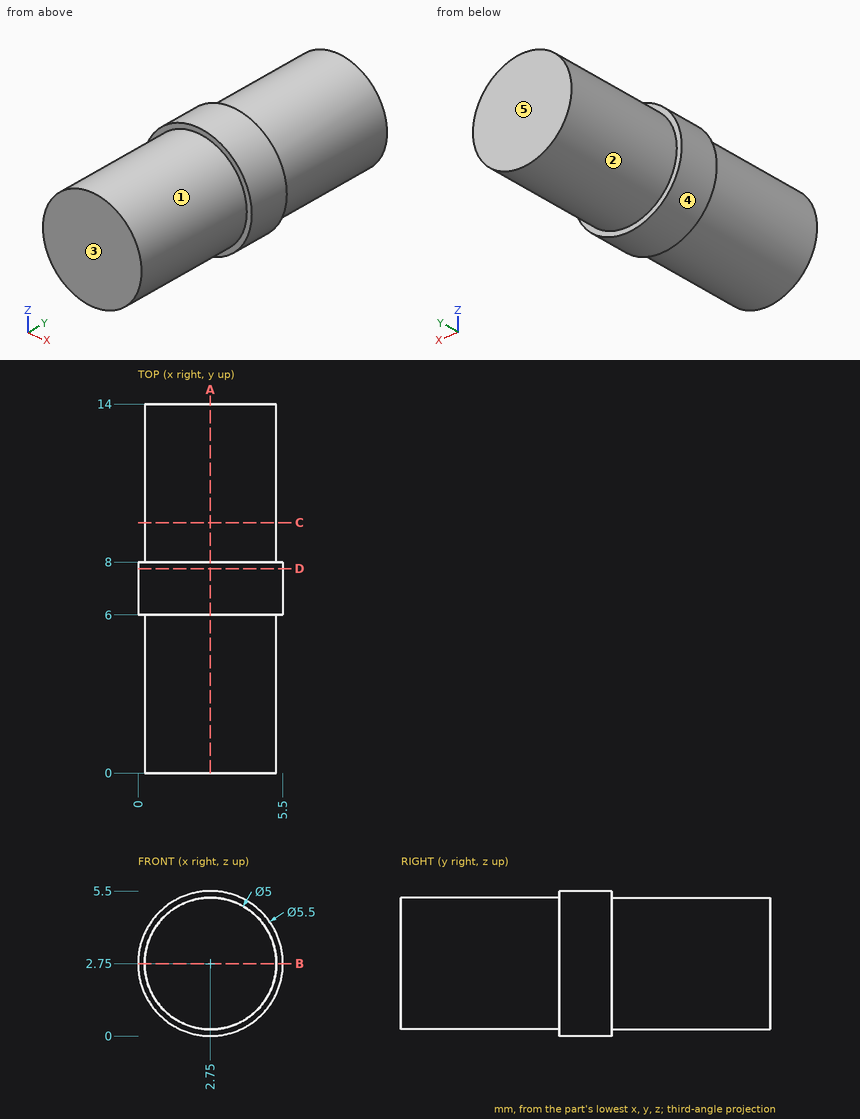
Verification items for this drawing (mm, ordinates from the low corner). A direction names the side the tool comes from. Give positions to 0.01 mm unless a question says otherwise; leave off trailing zeros. Loops run counter-clockwise (first coordinate to the right, second up) from the corner with the lowest first, then second, coordinate; pieces in that order, holes last. Notation, with made-up numbers: M 50.5,-18 L 65.5,-18 A18 ccw 65.5,-4 Z; hole C -19,49 d7. An arc over 180 degrees is marked long. Answer in a Markdown table with one row per item.
1) Tool access check on the marked faces 1, 2 and 3. Record the directions out of +Z, -Z, +X, -X, +Y, -Y that give a thin tool (end or side, any length) a straight path to the whole face; none if there is none.
Solutions:
| item | result |
|---|---|
| face 1 | -Y |
| face 2 | +Y |
| face 3 | +Z, -Z, +X, -X, -Y |
2) Mould release check, pull along Z, two halves, no side actions. Record for the marked faces 4 and 5: released by +Z, released by -Z, zero draft, split by the parting line, or undercut.
Solutions:
| item | result |
|---|---|
| face 4 | split by the parting line |
| face 5 | zero draft |
3) Cross-section at A-A (x = 2.75). Enter the section's corners in (y, z), plus the area to 3 significant figures.
Solutions:
| item | result |
|---|---|
| outline | M 0,0.25 L 6,0.25 L 6,0 L 8,0 L 8,0.25 L 14,0.25 L 14,5.25 L 8,5.25 L 8,5.5 L 6,5.5 L 6,5.25 L 0,5.25 Z |
| area | 71.0 mm^2 |
4) Thickness scan on line 1 (Z direction, x = 2.8, y = 8.5); line 2 (Z direction, x = 3.55, y = 6.25). Record the ranges inside material, lowest first.
Solutions:
| item | result |
|---|---|
| line 1 | z = 0.25 to 5.25 |
| line 2 | z = 0.12 to 5.38 |
5) Cross-section at C-C (y = 9.5). Enter the section's corners in (x, z), plus the area to 3 significant figures.
Solutions:
| item | result |
|---|---|
| outline | C 2.75,2.75 d5 |
| area | 19.6 mm^2 |
6) Cross-section at B-B (z = 2.75). Enter the section's corners in (x, y), plus the area to 3 significant figures.
Solutions:
| item | result |
|---|---|
| outline | M 0,6 L 0.25,6 L 0.25,0 L 5.25,0 L 5.25,6 L 5.5,6 L 5.5,8 L 5.25,8 L 5.25,14 L 0.25,14 L 0.25,8 L 0,8 Z |
| area | 71.0 mm^2 |
7) Cross-section at D-D (y = 7.75). Enter the section's corners in (x, z), plus the area to 3 significant figures.
Solutions:
| item | result |
|---|---|
| outline | C 2.75,2.75 d5.5 |
| area | 23.8 mm^2 |
